from build123d import *

# Parameters (mm, degrees)
F0_R     = 12.7
F0_R_2   = 6.35
F1_DEPTH = 19.05
F3_W     = 25.4
F3_H     = 6.35
F6_DEPTH = 19.051


with BuildPart() as f1:
    # F0 (on Top) → F1 (new body)
    with BuildSketch(Plane.XY):
        Circle(F0_R)
        Circle(F0_R_2, mode=Mode.SUBTRACT)
    extrude(amount=F1_DEPTH)

    # F3 (on offset) → F4 (join, up to the next surface of F1)
    with BuildSketch(Plane.YZ.offset(38.1)):
        with Locations((0, 3.175)):
            Rectangle(F3_W, F3_H)
    extrude(until=Until.NEXT, dir=(-1, 0, 0))

    # F5 (on face) → F6 (cut, through all)
    with BuildSketch(Plane(origin=(0, 0, 0), x_dir=(1, 0, 0), z_dir=(0, 0, -1))):
        Polygon((25.4, 12.7), (38.1, 0), (38.1, 12.7), align=None)
    extrude(amount=-F6_DEPTH, mode=Mode.SUBTRACT)


solid = f1.part
Could you check a few things on this model? Use its own coordinates, in mm. A direction names the side the tool comes from. Coordinates: 2 decimals unless noted, no trailing zeros. Order: outer loops, then holes, each group sorted by start corner. A loop starts at its lowest first (then second) coordinate and runs counter-clockwise, first axis right, second up.
Q1. Suppose I cut it at B-B on z = 1.75. Please give me the cut outline in (x, y).
Q2. Please list where these lines run through material, in increasing order: L1, parallel to Y at x = 0, z = 4; L2, parallel to X at y = -4.25, z = 11; L3, parallel to X at y = 2, z = 11.75.
Q3. Which directions (+Z, -Z, +X, -X, +Y, -Y) give clear straight access to the entire face, cutting with the end or side of a thin tool? Please do faces 1 (the cylindrical face through (-12.688, 0.558, 11.508)), 2 (the flat face through (38.1, 6, 3)).
Q4. Suppose I cut it at A-A on y = 5.75. Please give me the cut outline in (x, z).
Q5. Will these pins go through, and if not, where does the flat tip stop? pin 1 (5 mm diameter, centred on x = -6, z = 17, fed in from -Y); pin 2 (3 mm diameter, centred on x = -5, z = 6, fed in from +Y); pin 3 (6 mm diameter, centred on y = -8, z = 11, fed in from +X).
Q6. Suppose I cut it at D-D on y = 10. Please give me the cut outline in (x, z), and give its area (4 significant figures).
Q7. Thinking about a two-plate mould opening in X: for faces 3 (the flat face through (31.7, -6.4, 3.1)), 4 (the cylindrical face through (-1.38, -6.2, 9.39)), 5 (the flat face through (19, 12.7, 3)), which applies, released by +X, released by -X, zero draft, split by the parting line, or undercut?
Q8. Suppose I cut it at C-C on x = 17. Please give me the cut outline in (y, z), and give its area (3 significant figures).
Answer:
1. outline: (0, -12.7) - (25.4, -12.7) - (38.1, 0) - (38.1, 12.7) - (0, 12.7) arc R12.7 ccw to start; hole circle Ø12.7 at (0, 0)
2. L1: y = -12.7 to -6.35, 6.35 to 12.7
2. L2: x = -11.97 to -4.72, 4.72 to 11.97
2. L3: x = -12.54 to -6.03, 6.03 to 12.54
3. face 1: +Z
3. face 2: +Z, -Z, +X, +Y, -Y
4. outline: (-11.32, 0) - (-2.69, 0) - (-2.69, 19.05) - (-11.32, 19.05) - close; (2.69, 0) - (38.1, 0) - (38.1, 6.35) - (11.32, 6.35) - (11.32, 19.05) - (2.69, 19.05) - close
5. pin 1: stops at y = -12.21
5. pin 2: stops at y = 12.21
5. pin 3: stops at x = 11.67
6. outline: (-7.83, 0) - (38.1, 0) - (38.1, 6.35) - (7.83, 6.35) - (7.83, 19.05) - (-7.83, 19.05) - close
6. area: 490.5 mm2
7. face 3: released by +X
7. face 4: undercut
7. face 5: zero draft
8. outline: (-12.7, 0) - (12.7, 0) - (12.7, 6.35) - (-12.7, 6.35) - close
8. area: 161 mm2
